from build123d import *

# Parameters (mm, degrees)
F0_W     = 111.125
F0_H     = 9.0678
F1_DEPTH = 2.54
F2_R     = 0.633777
F3_DEPTH = 131.826


with BuildPart() as f1:
    # F0 (on Front) → F1 (new body)
    with BuildSketch(Plane.XZ):
        with Locations((28.219257, -22.19226)):
            Rectangle(F0_W, F0_H)
    extrude(amount=-F1_DEPTH)

    # F2 (on face) → F3 (cut)
    with BuildSketch(Plane.YZ.offset(83.781757)):
        with Locations((1.27, -22.19226)):
            Circle(F2_R)
    extrude(amount=-F3_DEPTH, mode=Mode.SUBTRACT)


solid = f1.part
Model file for the job. Use its own axes, mm. Coordinates: 2 decimals unless noted, no trailing zeros. Write each loop counter-clockwise with the first axis right and the second up, starting at its lowest first coordinate (ties: lowest second). Pieces come first, ordered by that corner, then holes. Notation, with made-up numbers: (58, -21) -> (89, -21) arc R22 cw to (89, -13) -> close; hole circle Ø4 at (48, -29.5). An arc over 180 degrees is marked (long way). One line per item, written item: value. Start each with the question number.
1) Pull direction X, two halves, no side cores. Call faces 1 (the face through (27, 0, -22)), 2 (the face through (83.782, 2.1, -22.3)), 3 (the face through (-27.343, 2.1, -22.3)): +X half, -X half, draft (parallel to the pull), parting line (faces both ways), or undercut.
2) Flat gauge pin, fed straight in: pin 1 Ø2 at (x, z) = (59, -23.5) entering from -Y. Where does the tip first touch, or does it go through?
3) Slice it at A-A on y = 1.27. Write the cut outline in (x, z).
4) Probe probe 1 along Z at (x, y) = (55.5, 1.27); probe 2 along Z at (x, y) = (-12, 1.7); probe 3 along Y at (x, z) = (45, -22.5). List the from-to ranges inside material, lowest first.
5) Slice it at B-B on x = 19. Write the cut outline in (y, z), then the cut area to 3 significant figures.
Answers follow:
1. face 1: draft
1. face 2: +X half
1. face 3: -X half
2. pin 1: y = 0
3. outline: (-27.34, -26.73) -> (83.78, -26.73) -> (83.78, -22.83) -> (-27.34, -22.83) -> close; (-27.34, -21.56) -> (83.78, -21.56) -> (83.78, -17.66) -> (-27.34, -17.66) -> close
4. probe 1: -26.73 to -22.83, -21.56 to -17.66
4. probe 2: -26.73 to -22.66, -21.73 to -17.66
4. probe 3: 0 to 0.72, 1.82 to 2.54
5. outline: (0, -26.73) -> (2.54, -26.73) -> (2.54, -17.66) -> (0, -17.66) -> close; hole circle Ø1.27 at (1.27, -22.19)
5. area: 21.8 mm2
